```python
from build123d import *

# Parameters (mm, degrees)
BOSS_EXTRUDE1_DEPTH = 3.175
SKETCH3_R           = 6.35
CUT_EXTRUDE1_DEPTH  = 4.1750001
SKETCH4_W           = 12.7
SKETCH4_H           = 12.7
CUT_EXTRUDE2_DEPTH  = 4.1750001
CUT_EXTRUDE3_DEPTH  = 4.1750001
SKETCH9_R           = 9.525
CUT_EXTRUDE5_DEPTH  = 5.08


with BuildPart() as part:
    # Sketch2 → Boss-Extrude1 (new body)
    with BuildSketch(Plane.XY):
        with BuildLine():
            add(Edge.make_bspline(
                [(318.77, 0.4016502), (318.651672051, 0.500810625), (317.887139521, 0.407183952), (316.525702267, 0.790429835), (314.029007456, 1.027310814), (310.665580368, 1.535686456), (306.332982445, 2.102999714), (301.108142881, 2.802187224), (295.00465514, 3.592552282), (288.066717306, 4.4725213), (280.334877508, 5.426678676), (271.857503414, 6.442111261), (262.686702585, 7.506224727), (252.87894916, 8.604531435), (242.494745532, 9.723621949), (231.598187206, 10.849597023), (220.25642858, 11.967923085), (208.539426289, 13.062902197), (196.51933871, 14.120159542), (184.270405083, 15.122019671), (171.867889749, 16.052147213), (159.388371015, 16.893273609), (146.908740176, 17.627811631), (134.505824677, 18.237204103), (122.256224526, 18.705201007), (110.2351092, 19.016534527), (98.516766738, 19.155997955), (87.173201506, 19.112523415), (76.274349541, 18.877713447), (65.887298252, 18.445615875), (56.075981931, 17.815100401), (46.900701285, 16.988064202), (38.417602501, 15.970966467), (30.678392783, 14.772461193), (23.72996987, 13.405065743), (17.613059426, 11.884241622), (12.362420389, 10.224818762), (8.00472945, 8.442252382), (4.553883407, 6.548602381), (2.01519229, 4.54013128), (0.389181285, 2.368249597), (-0.181372316, 0), (0.389181285, -2.368249597), (2.01519229, -4.54013128), (4.553883407, -6.548602381), (8.00472945, -8.442252382), (12.362420389, -10.224818762), (17.613059426, -11.884241622), (23.72996987, -13.405065743), (30.678392783, -14.772461193), (38.417602501, -15.970966467), (46.900701285, -16.988064202), (56.075981931, -17.815100401), (65.887298252, -18.445615875), (76.274349541, -18.877713447), (87.173201506, -19.112523415), (98.516766738, -19.155997955), (110.2351092, -19.016534527), (122.256224526, -18.705201007), (134.505824677, -18.237204103), (146.908740176, -17.627811631), (159.388371015, -16.893273609), (171.867889749, -16.052147213), (184.270405083, -15.122019671), (196.51933871, -14.120159542), (208.539426289, -13.062902197), (220.25642858, -11.967923085), (231.598187206, -10.849597023), (242.494745532, -9.723621949), (252.87894916, -8.604531435), (262.686702585, -7.506224727), (271.857503414, -6.442111261), (280.334877508, -5.426678676), (288.066717306, -4.4725213), (295.00465514, -3.592552282), (301.108142881, -2.802187224), (306.332982445, -2.102999714), (310.665580368, -1.535686456), (314.029007456, -1.027310814), (316.525702267, -0.790429835), (317.887139521, -0.407183952), (318.96162857, -0.538768719), (318.96162857, 0.241062861), (318.77, 0.4016502)],
                knots=[0, 0, 0, 0, 0.000762215, 0.003044706, 0.006832246, 0.012101176, 0.018817536, 0.026939455, 0.036414848, 0.047184629, 0.059180413, 0.072327874, 0.086544061, 0.10174058, 0.117823336, 0.134691452, 0.152240154, 0.17036129, 0.188941008, 0.207865435, 0.227016078, 0.246275696, 0.265524943, 0.284644966, 0.303520118, 0.322034575, 0.340078353, 0.357542593, 0.374325482, 0.390329891, 0.40546389, 0.419643801, 0.432793371, 0.444843817, 0.455737921, 0.465428653, 0.47388632, 0.481101634, 0.487101684, 0.491975368, 0.495930678, 0.499382808, 0.502834938, 0.506790248, 0.511663932, 0.517663982, 0.524879296, 0.533336963, 0.543027695, 0.553921799, 0.565972245, 0.579121815, 0.593301726, 0.608435725, 0.624440134, 0.641223023, 0.658687263, 0.676731041, 0.695245498, 0.71412065, 0.733240673, 0.75248992, 0.771749538, 0.790900181, 0.809824608, 0.828404326, 0.846525462, 0.864074164, 0.88094228, 0.897025036, 0.912221555, 0.926437743, 0.939585203, 0.951580988, 0.962350768, 0.971826161, 0.979948081, 0.98666444, 0.991933371, 0.99572091, 0.998003402, 0.998765616, 1, 1, 1, 1], degree=3))
        make_face()
    extrude(amount=BOSS_EXTRUDE1_DEPTH)

    # Sketch3 → Cut-Extrude1 (cut, through all)
    with BuildSketch(Plane.XY.offset(3.175)):
        with Locations((127, 0)):
            Circle(SKETCH3_R)
        Polygon((146.041832216, 17.654123083), (145.719448384, 11.304123083), (139.377616168, 11.626092244), (139.7, 17.976092244), (139.972135492, 23.336349817), (146.313967709, 23.014380656), align=None)
        Polygon((145.719448384, -11.304123083), (139.377616168, -11.626092244), (139.7, -17.976092244), (139.876824838, -21.459014187), (146.218657054, -21.137045026), (146.041832216, -17.654123083), align=None)
    extrude(amount=-CUT_EXTRUDE1_DEPTH, mode=Mode.SUBTRACT)

    # Sketch4 → Cut-Extrude2 (cut, through all)
    with BuildSketch(Plane.XY.offset(3.175)):
        with Locations((6.35, 0)):
            Rectangle(SKETCH4_W, SKETCH4_H)
    extrude(amount=-CUT_EXTRUDE2_DEPTH, mode=Mode.SUBTRACT)

    # Sketch5 → Cut-Extrude3 (cut, through all)
    with BuildSketch(Plane.XY.offset(3.175)):
        with BuildLine():
            Line((188.763328764, 17.093497057), (187.34983048, 15.089350861))
            ThreePointArc((187.34983048, 15.089350861), (183.094624601, 8.144494137), (183.023721428, 0))
            ThreePointArc((183.023721428, 0), (183.072311074, -8.06586998), (187.230894162, -14.977223407))
            Line((187.230894162, -14.977223407), (188.588975382, -18.075111724))
            add(Edge.make_bspline(
                [(188.588975382, -18.075111724), (191.824355535, -17.830310957), (199.841087156, -17.206236773), (212.516511905, -16.154636366), (226.466564745, -14.920704924), (239.970203835, -13.65677605), (252.944086016, -12.381118049), (265.308209748, -11.110630122), (276.986217406, -9.861474653), (287.906030173, -8.649252334), (298.000356614, -7.490870717), (307.207112828, -6.401010018), (315.468663619, -5.394751924), (322.736664519, -4.490202252), (328.958509167, -3.688972861), (334.117780822, -3.039413883), (338.123361689, -2.454274616), (341.095902765, -2.187108839), (342.718315982, -1.739066598), (343.996214648, -1.901995728), (344.002571846, -0.619693067), (342.723120546, -0.769943771), (341.105229436, -0.305837259), (338.135483436, -0.009211749), (334.135901144, 0.615614253), (328.983323498, 1.316295691), (322.769728908, 2.179175541), (315.511053915, 3.155743275), (307.259886312, 4.24386552), (298.064388673, 5.42495801), (287.982043821, 6.683368345), (277.074787054, 8.003801467), (265.409738858, 9.368683456), (253.058819828, 10.761699723), (240.098223582, 12.165931591), (226.607780172, 13.563687468), (212.670647531, 14.9358736), (200.006272506, 16.113099669), (191.996122671, 16.816629398), (188.763328764, 17.093497057)],
                knots=[0.797255798, 0.797255798, 0.797255798, 0.797255798, 0.809824608, 0.828404326, 0.846525462, 0.864074164, 0.88094228, 0.897025036, 0.912221555, 0.926437743, 0.939585203, 0.951580988, 0.962350768, 0.971826161, 0.979948081, 0.98666444, 0.991933371, 0.99572091, 0.998003402, 0.998765616, 1, 1.000762215, 1.003044706, 1.006832246, 1.012101176, 1.018817536, 1.026939455, 1.036414848, 1.047184629, 1.059180413, 1.072327874, 1.086544061, 1.10174058, 1.117823336, 1.134691452, 1.152240154, 1.17036129, 1.188941008, 1.201509818, 1.201509818, 1.201509818, 1.201509818], degree=3))
        make_face()
    extrude(amount=-CUT_EXTRUDE3_DEPTH, mode=Mode.SUBTRACT)

    # Sketch9 → Cut-Extrude5 (cut)
    with BuildSketch(Plane.XY.offset(3.175)):
        with Locations((165.1, 0)):
            Circle(SKETCH9_R)
    extrude(amount=-CUT_EXTRUDE5_DEPTH, mode=Mode.SUBTRACT)


solid = part.part
```
Part model, mm, in its own coordinate system. A direction names the side the tool comes from. Give positions to 0.01 mm unless a question says otherwise; leave off trailing zeros. Use one line per item in the form item = value.
Item 1: Slice it at A-A on z = 1.2. Count the separate pieces of the cut face and the enclosed holes in it, and give its area (3 significant figures).
Solution:
separate_pieces = 1
enclosed_holes = 2
area = 5,430 mm2
Item 2: Two-plate mould, pull along Y, no slides. Class faces 1 (the face through (95, 0, 3.175)), 2 (the face through (145.883, -14.524, 1.61)), 3 (the face through (133.057, 1.907, 1.61)): released by +Y, released by -Y, zero draft, split by the parting line, or undercut.
Solution:
face_1 = zero draft
face_2 = released by -Y
face_3 = undercut
Item 3: Pin check, flat tips, straight feed: pin 1 Ø1 at (x, z) = (8.5, 1.5) entering from +Y; pin 2 Ø1 at (y, z) = (2, 1.5) entering from -X; pin 3 Ø1.5 at (y, z) = (-9, 0.5) entering from +X. Stop position of each tip, or through.
Solution:
pin_1 = 8.81
pin_2 = 12.7
pin_3 = 183.65
Item 4: Probe probe 1 along X at (y, z) = (2, 0.4); probe 2 along X at (y, z) = (-1.5, 0.2); probe 3 along Y at (x, z) = (124, 1.1). List the from-to ranges inside material, lowest first. Write a range as from..to.
Solution:
probe_1 = 12.7..120.97, 133.03..155.79, 174.41..182.63
probe_2 = 12.7..120.83, 133.17..155.69, 174.51..182.7
probe_3 = -18.62..-5.6, 5.6..18.62
Item 5: Which spindle directions (+Z, -Z, +X, -X, +Y, -Y) get a long thin tool onto all of the face, cutting with end or side? Do faces 4 (the face through (139.537, 14.757, 1.61)), 5 (the face through (9, 6.35, 2)), 6 (the face through (145.883, 14.524, 1.61)). Say none if no direction does.
Solution:
face_4 = +Z, -Z
face_5 = +Z, -Z, -X
face_6 = +Z, -Z, +Y
